Can you work these out from the model? Positions are in its coordinate system, mm. A direction names the side the tool comes from. Coordinates: 2 decimals unless noted, no trailing zeros. Loops run counter-clockwise (first coordinate to the right, second up) from the corner with the lowest first, then second, coordinate; pieces in that order, holes last.
```python
from build123d import *

# Parameters (mm, degrees)
SKETCH1_R           = 16
SKETCH1_R_2         = 4
BOSS_EXTRUDE1_DEPTH = 12.5
BOSS_EXTRUDE2_START = 5
SKETCH1_3_R         = 16
BOSS_EXTRUDE2_DEPTH = 5
SKETCH2_R           = 16
BOSS_EXTRUDE3_DEPTH = 8
BOSS_EXTRUDE3_TAPER = 45
SKETCH4_R           = 8
BOSS_EXTRUDE4_DEPTH = 12


with BuildPart() as part:
    # Sketch1 → Boss-Extrude1 (new body)
    with BuildSketch(Plane.YZ):
        with Locations(Location((0, 0, 0), (0, 0, 270))):
            Circle(SKETCH1_R)
        with Locations(Location((0, 0, 0), (0, 0, 270))):
            Circle(SKETCH1_R_2, mode=Mode.SUBTRACT)
    extrude(amount=-BOSS_EXTRUDE1_DEPTH)

    # Sketch1_3 → Boss-Extrude2 (add)
    with BuildSketch(Plane.YZ.offset(BOSS_EXTRUDE2_START)):
        with Locations(Location((0, 0, 0), (0, 0, 270))):
            Circle(SKETCH1_3_R)
        with BuildLine():
            ThreePointArc((-4.453103796, -9.74483847), (-4.442785625, -9.66347175), (-4.436480838, -9.581696098))
            ThreePointArc((-4.436480838, -9.581696098), (-5.200182393, -8.091641748), (-6.872836595, -8.015945326))
            ThreePointArc((-6.872836595, -8.015945326), (-6.944603241, -8.055651196), (-7.014330689, -8.098837891))
            ThreePointArc((-7.014330689, -8.098837891), (-8.017688064, -8.608122706), (-9.107689918, -8.887394979))
            ThreePointArc((-9.107689918, -8.887394979), (-9.617215633, -8.333364784), (-10.093093531, -7.750178588))
            ThreePointArc((-10.093093531, -7.750178588), (-9.661540409, -6.711015969), (-9.014646736, -5.790350112))
            ThreePointArc((-9.014646736, -5.790350112), (-8.961976369, -5.727478496), (-8.912461189, -5.662093066))
            ThreePointArc((-8.912461189, -5.662093066), (-8.749343619, -3.995691347), (-10.1155453, -3.027706329))
            ThreePointArc((-10.1155453, -3.027706329), (-10.197385858, -3.022309054), (-10.27939281, -3.02094251))
            ThreePointArc((-10.27939281, -3.02094251), (-11.398810905, -2.906924208), (-12.466764806, -2.552563501))
            ThreePointArc((-12.466764806, -2.552563501), (-12.595873777, -1.811013243), (-12.680913477, -1.06312678))
            ThreePointArc((-12.680913477, -1.06312678), (-11.756054161, -0.422242789), (-10.714103032, 0.002533493))
            ThreePointArc((-10.714103032, 0.002533493), (-10.635802938, 0.026948711), (-10.558798085, 0.055184508))
            ThreePointArc((-10.558798085, 0.055184508), (-9.520650065, 1.368862824), (-10.146639845, 2.921808034))
            ThreePointArc((-10.146639845, 2.921808034), (-10.212570517, 2.970594857), (-10.280820345, 3.016080773))
            ThreePointArc((-10.280820345, 3.016080773), (-11.160891825, 3.717202186), (-11.867729954, 4.592688853))
            ThreePointArc((-11.867729954, 4.592688853), (-11.575430994, 5.286322206), (-11.242632993, 5.961460269))
            ThreePointArc((-11.242632993, 5.961460269), (-10.118103781, 6.000589494), (-9.011907317, 5.794612731))
            ThreePointArc((-9.011907317, 5.794612731), (-8.932837223, 5.772819893), (-8.852791194, 5.75494139))
            ThreePointArc((-8.852791194, 5.75494139), (-7.269217386, 6.298812721), (-6.956247932, 7.943668991))
            ThreePointArc((-6.956247932, 7.943668991), (-6.985336195, 8.020355891), (-7.018160061, 8.095519721))
            ThreePointArc((-7.018160061, 8.095519721), (-7.379468448, 9.161143151), (-7.500774695, 10.279794946))
            ThreePointArc((-7.500774695, 10.279794946), (-6.879870658, 10.705287707), (-6.234895971, 11.093325804))
            ThreePointArc((-6.234895971, 11.093325804), (-5.267726942, 10.518277011), (-4.448494704, 9.74694337))
            ThreePointArc((-4.448494704, 9.74694337), (-4.393758806, 9.685861548), (-4.33608565, 9.627545044))
            ThreePointArc((-4.33608565, 9.627545044), (-2.709859549, 9.228934084), (-1.557296451, 10.443471171))
            ThreePointArc((-1.557296451, 10.443471171), (-1.540306987, 10.523710598), (-1.527283546, 10.604688358))
            ThreePointArc((-1.527283546, 10.604688358), (-1.255115981, 11.696485895), (-0.752376468, 12.703138778))
            ThreePointArc((-0.752376468, 12.703138778), (-0.376352864, 12.719833477), (0, 12.7254))
            ThreePointArc((0, 12.7254), (0.376352864, 12.719833477), (0.752376468, 12.703138778))
            ThreePointArc((0.752376468, 12.703138778), (1.255115981, 11.696485895), (1.527283546, 10.604688358))
            ThreePointArc((1.527283546, 10.604688358), (1.540306987, 10.523710598), (1.557296451, 10.443471171))
            ThreePointArc((1.557296451, 10.443471171), (2.709859549, 9.228934084), (4.33608565, 9.627545044))
            ThreePointArc((4.33608565, 9.627545044), (4.393758806, 9.685861548), (4.448494704, 9.74694337))
            ThreePointArc((4.448494704, 9.74694337), (5.267726942, 10.518277011), (6.234895971, 11.093325804))
            ThreePointArc((6.234895971, 11.093325804), (6.879870658, 10.705287707), (7.500774695, 10.279794946))
            ThreePointArc((7.500774695, 10.279794946), (7.379468448, 9.161143151), (7.018160061, 8.095519721))
            ThreePointArc((7.018160061, 8.095519721), (6.985336195, 8.020355891), (6.956247932, 7.943668991))
            ThreePointArc((6.956247932, 7.943668991), (7.269217386, 6.298812721), (8.852791194, 5.75494139))
            ThreePointArc((8.852791194, 5.75494139), (8.932837223, 5.772819893), (9.011907317, 5.794612731))
            ThreePointArc((9.011907317, 5.794612731), (10.118103781, 6.000589494), (11.242632993, 5.961460269))
            ThreePointArc((11.242632993, 5.961460269), (11.575430994, 5.286322206), (11.867729954, 4.592688853))
            ThreePointArc((11.867729954, 4.592688853), (11.160891825, 3.717202186), (10.280820345, 3.016080773))
            ThreePointArc((10.280820345, 3.016080773), (10.212570517, 2.970594857), (10.146639845, 2.921808034))
            ThreePointArc((10.146639845, 2.921808034), (9.520650065, 1.368862824), (10.558798085, 0.055184508))
            ThreePointArc((10.558798085, 0.055184508), (10.635802938, 0.026948711), (10.714103032, 0.002533493))
            ThreePointArc((10.714103032, 0.002533493), (11.756054161, -0.422242789), (12.680913477, -1.06312678))
            ThreePointArc((12.680913477, -1.06312678), (12.595873777, -1.811013243), (12.466764806, -2.552563501))
            ThreePointArc((12.466764806, -2.552563501), (11.398810905, -2.906924208), (10.27939281, -3.02094251))
            ThreePointArc((10.27939281, -3.02094251), (10.197385858, -3.022309054), (10.1155453, -3.027706329))
            ThreePointArc((10.1155453, -3.027706329), (8.749343619, -3.995691347), (8.912461189, -5.662093066))
            ThreePointArc((8.912461189, -5.662093066), (8.961976369, -5.727478496), (9.014646736, -5.790350112))
            ThreePointArc((9.014646736, -5.790350112), (9.661540409, -6.711015969), (10.093093531, -7.750178588))
            ThreePointArc((10.093093531, -7.750178588), (9.617215633, -8.333364784), (9.107689918, -8.887394979))
            ThreePointArc((9.107689918, -8.887394979), (8.01768807, -8.608122703), (7.014330701, -8.098837886))
            ThreePointArc((7.014330701, -8.098837886), (6.944603253, -8.055651191), (6.872836606, -8.015945321))
            ThreePointArc((6.872836606, -8.015945321), (5.200182396, -8.091641744), (4.436480837, -9.5816961))
            ThreePointArc((4.436480837, -9.5816961), (4.442785625, -9.663471753), (4.453103796, -9.744838473))
            ThreePointArc((4.453103796, -9.744838473), (4.499555842, -10.869089), (4.300787703, -11.976603454))
            ThreePointArc((4.300787703, -11.976603454), (3.585159479, -12.209931886), (2.856987833, -12.400541346))
            ThreePointArc((2.856987833, -12.400541346), (2.091005912, -11.576303066), (1.522268135, -10.605409465))
            ThreePointArc((1.522268135, -10.605409465), (1.486958164, -10.531381002), (1.448050834, -10.459178321))
            ThreePointArc((1.448050834, -10.459178321), (1e-09, -9.618553067), (-1.448050833, -10.459178319))
            ThreePointArc((-1.448050833, -10.459178319), (-1.486958163, -10.531381001), (-1.522268135, -10.605409465))
            ThreePointArc((-1.522268135, -10.605409465), (-2.091005912, -11.576303066), (-2.856987833, -12.400541346))
            ThreePointArc((-2.856987833, -12.400541346), (-3.585159479, -12.209931886), (-4.300787703, -11.976603454))
            ThreePointArc((-4.300787703, -11.976603454), (-4.499555842, -10.869088998), (-4.453103796, -9.74483847))
        make_face(mode=Mode.SUBTRACT)
    extrude(amount=-BOSS_EXTRUDE2_DEPTH)

    # Sketch2 → Boss-Extrude3 (add)
    with BuildSketch(Plane(origin=(-12.5, 0, 0), x_dir=(0, -1, 0), z_dir=(-1, 0, 0))):
        with Locations(Location((0, 0, 0), (0, 0, 270))):
            Circle(SKETCH2_R)
    extrude(amount=BOSS_EXTRUDE3_DEPTH, taper=BOSS_EXTRUDE3_TAPER)

    # Sketch4 → Boss-Extrude4 (add)
    with BuildSketch(Plane(origin=(-20.5, 0, 0), x_dir=(0, -1, 0), z_dir=(-1, 0, 0))):
        with Locations(Location((0, 0, 0), (0, 0, 90))):
            Circle(SKETCH4_R)
        with BuildLine():
            Line((-1.19, 3.818887272), (-1.19, 5.19))
            Line((-1.19, 5.19), (1.19, 5.19))
            Line((1.19, 5.19), (1.19, 3.818887272))
            ThreePointArc((1.19, 3.818887272), (3.221800739, 2.370653918), (4, 0))
            ThreePointArc((4, 0), (-2.370653918, -3.221800739), (-1.19, 3.818887272))
        make_face(mode=Mode.SUBTRACT)
    extrude(amount=BOSS_EXTRUDE4_DEPTH)


solid = part.part
```
Item 1: I need wall thicknesses on line 1 along Y through (x, z) = (-23, 0); line 2 along Z through (x, y) = (0.5, 7); line 3 along Z through (x, y) = (2, 11). Which ranges of each line are inside material? Lowest first, please.
Results are:
line 1: y = -8 to -4, 4 to 8
line 2: z = -14.39 to -8.09, 6.73 to 8.06, 10.63 to 14.39
line 3: z = -11.62 to -2.98, -0.09 to 3.56, 5.99 to 11.62
Item 2: Suppose I cut it at B-B, the plane x = -11. Please give me the cut outline in (y, z).
Results are:
outline: circle Ø32 at (0, 0); hole circle Ø8 at (0, 0)
Item 3: On a 3-axis mill with a long thin cutter (end or side, diameter ignored), from which of +Z, -Z, +X, -X, +Y, -Y can I reach the whole of each face in a straight line? I mean faces 5 (the face through (2.54, 9.62, -8.33)), 6 (the face through (-26, -1.19, 5)). Say none if no direction works.
Results are:
face 5: +X
face 6: -X
Item 4: We'd pull the mould along Z, two halves only. Please class faces 1 (the face through (5, 0, -10)), 2 (the face through (-26.42, -7.81, -1.73)), 3 (the face through (2.535, -9.669, -6.725)), 4 (the face through (2.5, -8, -8.6)): +Z half, -Z half, draft (parallel to the pull), parting line (faces both ways), or undercut.
Results are:
face 1: draft
face 2: parting line
face 3: undercut
face 4: undercut
Item 5: Suppose I cut it at A-A, the plane x = -25.5. Please give me the cut outline in (y, z), plus the area to 3 significant figures.
Results are:
outline: circle Ø16 at (0, 0); hole (-1.19, 3.82) arc R4 ccw (long way) to (1.19, 3.82) - (1.19, 5.19) - (-1.19, 5.19) - close
area: 148 mm2
Item 6: I'm going to push flat-ended pins straight in: P1, Ø12, axis at x = -24, y = 4, coming from the +Z side; P2, Ø1.5, axis at x = -24.5, z = 4.5, coming from the +Y side; P3, Ø5, axis at y = 0, z = 0, coming from the +X side. Where does each tip first touch, or does it pass through?
Results are:
P1: stops at z = 10
P2: stops at y = 7.07
P3: stops at x = -12.5
